```python
from build123d import *

# Parameters (mm, degrees)
SKETCH1_R           = 5
BOSS_EXTRUDE1_DEPTH = 4
SKETCH2_R           = 5.5
BOSS_EXTRUDE2_DEPTH = 1
SKETCH3_R           = 2.05
CUT_EXTRUDE1_DEPTH  = 6
CHAMFER1_SIZE       = 0.5


with BuildPart() as part:
    # Sketch1 → Boss-Extrude1 (new body)
    with BuildSketch(Plane.XY):
        Circle(SKETCH1_R)
    extrude(amount=BOSS_EXTRUDE1_DEPTH)

    # Sketch2 → Boss-Extrude2 (add)
    with BuildSketch(Plane.XY):
        Circle(SKETCH2_R)
    extrude(amount=-BOSS_EXTRUDE2_DEPTH)

    # Sketch3 → Cut-Extrude1 (cut, through all)
    with BuildSketch(Plane.XY.offset(4)):
        Circle(SKETCH3_R)
    extrude(amount=-CUT_EXTRUDE1_DEPTH, mode=Mode.SUBTRACT)

    # Chamfer1
    chamfer1_edges = [part.edges().sort_by_distance(p)[0] for p in [
        (-2.05, 0, -1),
        (-2.05, 0, 4),
        (-5, 0, 4),
        (-5.5, 0, -1),
    ]]
    chamfer(chamfer1_edges, length=CHAMFER1_SIZE)


solid = part.part
```
Here's how the part is built. I have some questions about the finished solid (model axes, mm). A direction names the side the tool comes from. Coordinates: 2 decimals unless noted, no trailing zeros. Write each loop counter-clockwise with the first axis right and the second up, starting at its lowest first coordinate (ties: lowest second). Pieces come first, ordered by that corner, then holes. Notation, with made-up numbers: (64.5, 22) - (116.5, 22) arc R13 ccw to (116.5, 31) - close; hole circle Ø7 at (-39, 9.25). An arc over 180 degrees is marked (long way). One line per item, written item: value.
1) On a 3-axis mill with a long thin cutter (end or side, diameter ignored), from which of +Z, -Z, +X, -X, +Y, -Y can I reach the whole of each face in a straight line? I mean faces 4 (the flat face through (2, -2, -1)), 5 (the cylindrical face through (-1.08, -4.88, 1.73)). Say none if no direction works.
Model answer:
face 4: -Z, +X, -X, +Y, -Y
face 5: +Z
2) I'm going to push flat-ended pins straight in: P1, Ø1, axis at x = 4, z = 3, coming from the -Y side; P2, Ø1.5, axis at y = 3, z = 0.5, coming from the -X side. Where does each tip first touch, or does it pass through?
Model answer:
P1: stops at y = -3.57
P2: stops at x = -4.93
3) I need wall thicknesses on line 1 along Y through (x, z) = (0, 1.75); line 2 along X through (y, z) = (-1.5, 0.7); line 3 along X through (y, z) = (0.75, 0.6). Which ranges of each line are inside material? Lowest first, please.
Model answer:
line 1: y = -5 to -2.05, 2.05 to 5
line 2: x = -4.77 to -1.4, 1.4 to 4.77
line 3: x = -4.94 to -1.91, 1.91 to 4.94
4) Suppose I cut it at C-C on z = 0.4. Write out the boundary of the cut face in (x, y).
Model answer:
outline: circle Ø10 at (0, 0); hole circle Ø4.1 at (0, 0)
5) We'd pull the mould along Y, two halves only. Please class faces 1 (the cylindrical face through (-1.19, -5.37, -0.25)), 2 (the flat face through (1.6, -4.9, 0)), 3 (the cylindrical face through (-0.267, 2.033, 1.528)): pulls with the +Y half, pulls with the -Y half, needs draft (parallel to the pull), parting line crosses it, or undercut.
Model answer:
face 1: parting line crosses it
face 2: needs draft
face 3: undercut
6) Suppose I cut it at A-A on x = 0. Write out the boundary of the cut face in (y, z), and give its area (3 significant figures).
Model answer:
outline: (-5.5, -0.5) - (-5, -1) - (-2.55, -1) - (-2.05, -0.5) - (-2.05, 3.5) - (-2.55, 4) - (-4.5, 4) - (-5, 3.5) - (-5, 0) - (-5.5, 0) - close; (2.05, -0.5) - (2.55, -1) - (5, -1) - (5.5, -0.5) - (5.5, 0) - (5, 0) - (5, 3.5) - (4.5, 4) - (2.55, 4) - (2.05, 3.5) - close
area: 29.5 mm²
